Source: CAD feature listing. Evaluate the final solid. Frame: model axes, mm. A direction names the side the tool comes from. Coordinates: 2 decimals unless noted, no trailing zeros. Loops run counter-clockwise (first coordinate to the right, second up) from the corner with the lowest first, then second, coordinate; pieces in that order, holes last. Notation, with made-up numbers: (29.25, 13) - (61.25, 13) arc R24 cw to (61.25, 52) - close; hole circle Ø4 at (-11, -13.75). An arc over 180 degrees is marked (long way). Write item = value, one per line. Start each with the question number.
from build123d import *

# Parameters (mm, degrees)
CROQUIS1_W              = 100
CROQUIS1_H              = 95
SALIENTE_EXTRUIR1_DEPTH = 40
CROQUIS3_W              = 20
CROQUIS3_H              = 46
CORTAR_EXTRUIR1_DEPTH   = 30
CROQUIS4_W              = 96
CROQUIS4_H              = 46
CORTAR_EXTRUIR2_DEPTH   = 38
CROQUIS5_W              = 65
CROQUIS5_H              = 67
CORTAR_EXTRUIR3_DEPTH   = 5
CROQUIS7_W              = 69
CROQUIS7_H              = 1.7
CORTAR_EXTRUIR4_DEPTH   = 46
CROQUIS9_W              = 5
CROQUIS9_H              = 15
CORTAR_EXTRUIR6_DEPTH   = 10
CROQUIS10_R             = 2.5
CORTAR_EXTRUIR8_DEPTH   = 143.302494708
CROQUIS11_W             = 46
CROQUIS11_H             = 30
CORTAR_EXTRUIR9_DEPTH   = 131.479883507
CROQUIS12_W             = 13.5
CROQUIS12_H             = 46
CROQUIS12_W_2           = 15.5
CORTAR_EXTRUIR10_DEPTH  = 144.614066163
CORTAR_EXTRUIR13_DEPTH  = 2
CORTAR_EXTRUIR14_DEPTH  = 2
CORTAR_EXTRUIR15_DEPTH  = 2
CROQUIS16_W             = 58
CROQUIS16_H             = 18
SALIENTE_EXTRUIR2_DEPTH = 16
CROQUIS17_W             = 53
CROQUIS17_H             = 13
CORTAR_EXTRUIR16_DEPTH  = 16


with BuildPart() as part:
    # Croquis1 → Saliente-Extruir1 (new body)
    with BuildSketch(Plane(origin=(0, 0, 0), x_dir=(1, 0, 0), z_dir=(0, 1, 0))):
        with Locations((50, 47.5)):
            Rectangle(CROQUIS1_W, CROQUIS1_H)
    extrude(amount=SALIENTE_EXTRUIR1_DEPTH)

    # Croquis3 → Cortar-Extruir1 (cut)
    with BuildSketch(Plane.XZ):
        with Locations((90, -72)):
            Rectangle(CROQUIS3_W, CROQUIS3_H)
        with Locations((10, -72)):
            Rectangle(CROQUIS3_W, CROQUIS3_H)
    extrude(amount=-CORTAR_EXTRUIR1_DEPTH, mode=Mode.SUBTRACT)

    # Croquis4 → Cortar-Extruir2 (cut)
    with BuildSketch(Plane(origin=(0, 40, 0), x_dir=(1, 0, 0), z_dir=(0, 1, 0))):
        with Locations((50, 25)):
            Rectangle(CROQUIS4_W, CROQUIS4_H)
    extrude(amount=-CORTAR_EXTRUIR2_DEPTH, mode=Mode.SUBTRACT)

    # Croquis5 → Cortar-Extruir3 (cut)
    with BuildSketch(Plane(origin=(0, 40, 0), x_dir=(1, 0, 0), z_dir=(0, 1, 0))):
        with Locations((51, 59.5)):
            Rectangle(CROQUIS5_W, CROQUIS5_H)
    extrude(amount=-CORTAR_EXTRUIR3_DEPTH, mode=Mode.SUBTRACT)

    # Croquis7 → Cortar-Extruir4 (cut)
    with BuildSketch(Plane.XY.offset(-48)):
        with Locations((51, 37)):
            Rectangle(CROQUIS7_W, CROQUIS7_H)
    extrude(amount=-CORTAR_EXTRUIR4_DEPTH, mode=Mode.SUBTRACT)

    # Croquis9 → Cortar-Extruir6 (cut)
    with BuildSketch(Plane(origin=(0, 40, 0), x_dir=(1, 0, 0), z_dir=(0, 1, 0))):
        with Locations((8.5, 77.5)):
            Rectangle(CROQUIS9_W, CROQUIS9_H)
        with Locations((91.5, 77.5)):
            Rectangle(CROQUIS9_W, CROQUIS9_H)
    extrude(amount=-CORTAR_EXTRUIR6_DEPTH, mode=Mode.SUBTRACT)

    # Croquis10 → Cortar-Extruir8 (cut, through all)
    with BuildSketch(Plane(origin=(0, 35, 0), x_dir=(1, 0, 0), z_dir=(0, 1, 0))):
        with Locations(Location((50, 72, 0), (0, 0, 270))):
            Circle(CROQUIS10_R)
    extrude(amount=-CORTAR_EXTRUIR8_DEPTH, mode=Mode.SUBTRACT)

    # Croquis11 → Cortar-Extruir9 (cut, through all)
    with BuildSketch(Plane(origin=(80, 0, 0), x_dir=(0, 0, -1), z_dir=(1, 0, 0))):
        with Locations((72, 15)):
            Rectangle(CROQUIS11_W, CROQUIS11_H)
    extrude(amount=-CORTAR_EXTRUIR9_DEPTH, mode=Mode.SUBTRACT)

    # Croquis12 → Cortar-Extruir10 (cut, through all)
    with BuildSketch(Plane(origin=(0, 40, 0), x_dir=(1, 0, 0), z_dir=(0, 1, 0))):
        with Locations((93.25, 72)):
            Rectangle(CROQUIS12_W, CROQUIS12_H)
        with Locations((7.75, 72)):
            Rectangle(CROQUIS12_W_2, CROQUIS12_H)
    extrude(amount=-CORTAR_EXTRUIR10_DEPTH, mode=Mode.SUBTRACT)

    # Croquis14 → Cortar-Extruir13 (cut)
    with BuildSketch(Plane(origin=(100, 0, 0), x_dir=(0, 0, -1), z_dir=(1, 0, 0))):
        Polygon((19, 25), (29, 25), (29, 2), (48, 2), (48, 40), (0, 40), (0, 2), (19, 2), align=None)
    extrude(amount=-CORTAR_EXTRUIR13_DEPTH, mode=Mode.SUBTRACT)

    # Croquis15 → Cortar-Extruir14 (cut)
    with BuildSketch(Plane.ZY):
        Polygon((-48, 2), (-48, 40), (0, 40), (0, 2), (-19, 2), (-19, 25), (-29, 25), (-29, 2), align=None)
    extrude(amount=-CORTAR_EXTRUIR14_DEPTH, mode=Mode.SUBTRACT)

    # Croquis13 → Cortar-Extruir15 (cut)
    with BuildSketch(Plane.XY):
        Polygon((2, 40), (98, 40), (98, 2), (92.75, 2), (92.75, 25), (67.75, 25), (67.75, 2), (62.5, 2), (62.5, 25), (37.5, 25), (37.5, 2), (32.25, 2), (32.25, 25), (7.25, 25), (7.25, 2), (2, 2), align=None)
    extrude(amount=-CORTAR_EXTRUIR15_DEPTH, mode=Mode.SUBTRACT)

    # Croquis16 → Saliente-Extruir2 (add)
    with BuildSketch(Plane(origin=(0, 2, 0), x_dir=(1, 0, 0), z_dir=(0, 1, 0))):
        with Locations((50, 39)):
            Rectangle(CROQUIS16_W, CROQUIS16_H)
    extrude(amount=SALIENTE_EXTRUIR2_DEPTH)

    # Croquis17 → Cortar-Extruir16 (cut)
    with BuildSketch(Plane(origin=(0, 18, 0), x_dir=(1, 0, 0), z_dir=(0, 1, 0))):
        with Locations((50, 39)):
            Rectangle(CROQUIS17_W, CROQUIS17_H)
    extrude(amount=-CORTAR_EXTRUIR16_DEPTH, mode=Mode.SUBTRACT)


solid = part.part
Item 1: Cut plane A-A (y = 11.5). State how many separate pieces and enclosed holes the cut face has, then the cut area to 3 significant figures.
Item 2: Cut plane C-C (y = 20). Return the cut outline in (x, z).
Item 3: Reachability of faces 1 (the flat face through (50, 10, -45.5)), 2 (the flat face through (15.5, 35, -72)), 3 (the flat face through (50, 18, -46)) from +Z, -Z, +X, -X, +Y, -Y: full face, straight path, thin tool, end or side. Return the list, or none.
Item 4: Cut plane D-D (z = -72). Return the cut outline in (x, y), then the cut area to 3 significant figures.
Item 5: Draft query along X for faces 4 (the flat face through (21, 10, -39)), 5 (the flat face through (51, 35, -66)), 6 (the flat face through (50, 10, -30)), 7 (the flat face through (86.5, 35, -72)). Return one class per face: released by +X, released by -X, zero draft, split by the parting line, or undercut.
Item 6: Cut plane B-B (x = 50). Return the cut outline in (y, z), then the cut area to 3 significant figures.
Item 7: First-contact query: pin 1 (1.7 mm diameter, centred on y = 39.5, z = -78.5, fed in from -X); pin 2 (8 mm diameter, centred on y = 11, z = -39, fed in from +X); pin 3 (1.5 mm diameter, centred on x = 40, y = 30, fed in from +Z). Flat tips, straight axial feed; report the tip coordinate or a pass-through.
Item 8: Material intervals for L1, parallel to X at y = 31.1, z = -72; L2, parallel to Z at x = 29, y = 9; L3, parallel to X at y = 8.5, z = -22, sorted ascending. Write a range as [from, to].
Responses:
q1.separate_pieces = 6
q1.enclosed_holes = 1
q1.area = 645 mm2
q2.outline = (0, -49) - (100, -49) - (100, -48) - (0, -48) - close; (0, -29) - (2, -29) - (2, -19) - (0, -19) - close; (7.25, -2) - (32.25, -2) - (32.25, 0) - (7.25, 0) - close; (37.5, -2) - (62.5, -2) - (62.5, 0) - (37.5, 0) - close; (67.75, -2) - (92.75, -2) - (92.75, 0) - (67.75, 0) - close; (98, -29) - (100, -29) - (100, -19) - (98, -19) - close
q3.face_1 = +Y
q3.face_2 = -Z, -X, +Y, -Y
q3.face_3 = +X, -X, +Y
q4.outline = (15.5, 30) - (47.5, 30) - (47.5, 35) - (18.5, 35) - (18.5, 36.15) - (16.5, 36.15) - (16.5, 37.85) - (18.5, 37.85) - (18.5, 40) - (15.5, 40) - close; (52.5, 30) - (86.5, 30) - (86.5, 40) - (83.5, 40) - (83.5, 37.85) - (85.5, 37.85) - (85.5, 36.15) - (83.5, 36.15) - (83.5, 35) - (52.5, 35) - close
q4.area = 353 mm2
q5.face_4 = released by -X
q5.face_5 = undercut
q5.face_6 = zero draft
q5.face_7 = released by +X
q6.outline = (0, -49) - (30, -49) - (30, -69.5) - (35, -69.5) - (35, -48) - (18, -48) - (18, -45.5) - (2, -45.5) - (2, -32.5) - (18, -32.5) - (18, -30) - (2, -30) - (2, -2) - (25, -2) - (25, 0) - (0, 0) - close; (30, -95) - (40, -95) - (40, -93) - (37.85, -93) - (37.85, -94) - (36.15, -94) - (36.15, -93) - (35, -93) - (35, -74.5) - (30, -74.5) - close
q6.area = 470 mm2
q7.pin_1 = 15.5
q7.pin_2 = 79
q7.pin_3 = -48
q8.L1 = [15.5, 47.5], [52.5, 86.5]
q8.L2 = [-49, -45.5], [-32.5, -30], [-2, 0]
q8.L3 = [0, 2], [98, 100]
